Autodesk Inventor part; units mm, degrees
ref_plane "YZ Plane" through (0, 0, 0) normal (1, 0, 0) x (0, 1, 0)
ref_plane "XZ Plane" through (0, 0, 0) normal (0, 1, 0) x (-1, 0, 0)
ref_plane "XY Plane" through (0, 0, 0) normal (0, 0, 1) x (1, 0, 0)
sketch "Sketch1" plane through (0, 0, 0) normal (0, 1, 0) x (-1, 0, 0)
  line L0 (-75, 47.5) -> (75, 47.5)
  line L1 (75, 47.5) -> (75, -47.5)
  line L2 (75, -47.5) -> (-75, -47.5)
  line L3 (-75, -47.5) -> (-75, 47.5)
  line L4 (-75, 47.5) -> (75, -47.5) construction
  line L5 (75, 47.5) -> (-75, -47.5) construction
  point P0 (0, 0)
  dimension "d0" = 150
  dimension "d1" = 95
extrude "Extrusion1" add sketch "Sketch1" along normal blind 3
sketch "Sketch4" plane through (0, 3, 0) normal (0, 1, 0) x (1, 0, 0)
  line L0 (75, 47.5) -> (-75, 47.5)
  line L1 (-10, 47.5) -> (10, 47.5)
  line L2 (10, 47.5) -> (10, 27.5)
  line L3 (-10, 47.5) -> (-10, 27.5)
  line L4 (-10, 27.5) -> (10, 27.5)
  line L5 (-13, 47.5) -> (-7, 47.5)
  line L6 (7, 47.5) -> (13, 47.5)
  line L7 (-10, 47.5) -> (-10, 42.5)
  line L8 (10, 47.5) -> (10, 42.5)
  line L9 (-10, 42.5) -> (-10, 39.5)
  line L10 (10, 42.5) -> (10, 39.5)
  line L11 (-10, 27.5) -> (-10, 30.5)
  line L12 (10, 27.5) -> (10, 30.5)
  circle A0 centre (-10, 30.5) radius 3
  circle A1 centre (10, 30.5) radius 3
  circle A2 centre (-10, 39.5) radius 3
  circle A3 centre (10, 39.5) radius 3
  line L13 (-13, 39.5) -> (-13, 30.5)
  line L14 (-7, 39.5) -> (-7, 30.5)
  line L15 (7, 39.5) -> (7, 30.5)
  line L16 (13, 39.5) -> (13, 30.5)
  line L17 (-10, 27.5) -> (-7, 27.5)
  line L18 (-7, 27.5) -> (-7, 47.5)
  line L19 (-7, 47.5) -> (-10, 47.5)
  line L20 (-10, 47.5) -> (-10, 27.5)
  line L21 (-10, 47.5) -> (-13, 47.5)
  line L22 (-13, 47.5) -> (-13, 27.5)
  line L23 (-13, 27.5) -> (-10, 27.5)
  line L24 (-10, 27.5) -> (-10, 47.5)
  line L25 (10, 27.5) -> (7, 27.5)
  line L26 (7, 27.5) -> (7, 47.5)
  line L27 (7, 47.5) -> (10, 47.5)
  line L28 (10, 47.5) -> (10, 27.5)
  line L29 (10, 27.5) -> (13, 27.5)
  line L30 (13, 27.5) -> (13, 47.5)
  line L31 (13, 47.5) -> (10, 47.5)
  line L32 (10, 47.5) -> (10, 27.5)
  point P0 (0, 0)
  point P1 (0, 47.5)
  point P2 (7, 47.5)
  point P3 (7, 39.5)
  point P4 (-7, 39.5)
  point P5 (-7, 47.5)
  point P6 (-13, 47.5)
  point P7 (-13, 39.5)
  dimension "d14" = 20
  dimension "d15" = 20
  dimension "d16" = 6
  dimension "d17" = 6
  dimension "d18" = 5
  dimension "d19" = 5
  dimension "d20" = 3
  dimension "d21" = 3
  dimension "d22" = 3
  dimension "d23" = 3
extrude "Extrusion3" cut sketch "Sketch4" against normal through all contours A3 L2 | L16 A1 L2 A3 | L2 A3 | L2 A1 L15 A3 | A1 L2 | L2 A1 | A2 L3 | L14 A0 L3 A2 | L3 A2 | L3 A0 L13 A2 | A0 L3 | L3 A0
extrude "Extrusion5" cut sketch "Sketch4" against normal blind 1.2 contours L30 A3 L2 L0 | L2 A3 L26 L0 | L18 A2 L3 L0 | L3 A2 L22 L0
sketch "Sketch6" plane through (0, 3, 0) normal (0, 1, 0) x (1, 0, 0)
  line L0 (75, 47.5) -> (-75, 47.5)
  line L1 (0, 47.5) -> (0, 22.5)
  line L2 (0, 22.5) -> (0, -20.7)
  line L3 (0, -20.7) -> (0, 0.9)
  line L4 (0, 0.9) -> (-53.4, 0.9)
  line L5 (-53.4, -15.1) -> (-53.4, 16.9)
  circle A0 centre (-53.4, 16.9) radius 3
  circle A1 centre (-53.4, -15.1) radius 3
  line L6 (-19, 0.9) -> (19, 0.9)
  circle A2 centre (19, 0.9) radius 2.5
  circle A3 centre (-19, 0.9) radius 2.5
  line L7 (-19, 0.9) -> (-17, 0.9)
  line L8 (19, 0.9) -> (17, 0.9)
  circle A4 centre (17, 0.9) radius 2.5
  circle A5 centre (-17, 0.9) radius 2.5
  line L9 (-19, 3.4) -> (-17, 3.4)
  line L10 (-19, -1.6) -> (-17, -1.6)
  line L11 (17, 3.4) -> (19, 3.4)
  line L12 (17, -1.6) -> (19, -1.6)
  point P0 (0, 0)
  dimension "d40" = 25
  dimension "d41" = 43.2
  dimension "d42" = 53.4
  dimension "d43" = 32
  dimension "d44" = 6
  dimension "d45" = 6
  dimension "d46" = 38
  dimension "d47" = 5
  dimension "d48" = 5
  dimension "d49" = 2
  dimension "d50" = 2
  dimension "d51" = 5
  dimension "d52" = 5
extrude "Extrusion6" cut sketch "Sketch6" against normal through all
sketch "Sketch7" plane through (0, 3, 0) normal (0, 1, 0) x (1, 0, 0)
  line L0 (75, 47.5) -> (-75, 47.5)
  line L1 (-75, -47.5) -> (75, -47.5)
  line L2 (75, 47.5) -> (35, 47.5)
  line L3 (35, 47.5) -> (35, -47.5)
  line L4 (35, -47.5) -> (75, -47.5)
  line L5 (75, -47.5) -> (75, 47.5)
  point P0 (0, 0)
  point P1 (75, -47.5)
  dimension "d55" = 40
extrude "Extrusion7" cut sketch "Sketch7" against normal through all
sketch "Sketch8" plane through (0, 3, 0) normal (0, 1, 0) x (1, 0, 0)
  line L0 (-75, -47.5) -> (35, -47.5)
  line L1 (7, 47.5) -> (-7, 47.5)
  line L2 (0, 47.5) -> (0, -42.5)
  circle A0 centre (0, -42.5) radius 25
  circle A1 centre (0, -42.5) radius 20
  line L3 (0, -42.5) -> (-20, -42.5)
  circle A2 centre (-20, -42.5) radius 1.5
  circle A3 centre (-10, -59.8205) radius 1.5
  circle A4 centre (10, -59.8205) radius 1.5
  circle A5 centre (20, -42.5) radius 1.5
  circle A6 centre (10, -25.1795) radius 1.5
  circle A7 centre (-10, -25.1795) radius 1.5
  circle A8 centre (0, -42.5) radius 17
  line L4 (-17, -42.5) -> (-17, -47.5)
  line L5 (17, -42.5) -> (17, -47.5)
  point P0 (0, 0)
  dimension "d60" = 90
  dimension "d61" = 50
  dimension "d62" = 40
  dimension "d63" = 20
  dimension "d64" = 3
  dimension "d67" = 360
  dimension "d69" = 34
extrude "Extrusion8" cut sketch "Sketch8" against normal through all contours L4 A8 L0 | A2 A1 | A1 L3 A2 | A8 L3 L2 L0 | A8 L2 L3 | A1 A2 L3 | A6 A1 | A1 A6 | A7 A1 | A1 A7 | L0 A8 L5 | A5 A1 | A1 A5
fillet "Fillet1" radius 10 4 edges at (35, 1.5, 47.5) (35, 1.5, -47.5) (-75, 1.5, 47.5) (-75, 1.5, -47.5)
properties part number "TopMount"
Check sheet for the modelled part. Datum: model origin and axes. Units: mm. A direction names the side the tool comes from. Give positions to 0.01 mm unless a question says otherwise; leave off trailing zeros. Write each loop counter-clockwise with the first axis right and the second up, starting at its lowest first coordinate (ties: lowest second). Pieces come first, ordered by that corner, then holes. Notation, with made-up numbers: (87.25, 47.25) - (126.25, 47.25) arc R26 ccw to (126.25, 86.25) - close; hole circle Ø8 at (-36.5, -3). An arc over 180 degrees is marked (long way). Answer as a JSON object with one key per item and string values. Group by question number.
1) Access from +Z, -Z, +X, -X, +Y, -Y to the whole of each face (thin tool, end or side, straight path). Record for faces 1 (the face through (-14.5, 1.5, -0.8)), 2 (the face through (-7, 2, -37)), 3 (the face through (0.374, 1.521, 25.504)).
2) Thickness scan on probe 1 along X at (y, z) = (2.2, -1); probe 2 along X at (y, z) = (2.3, -16.9); probe 3 along Z at (x, y) = (-53.4, 1.5). Record the ranges inside material, lowest first. Write a range as from..to.
3) Sectioned sample at A-A (x = -53.4). Record the cut outline in (y, z).
4) Release check for a two-part mould opening along X. For faces 4 (the face through (20, 2, 44)), 5 (the face through (-71.99, 1.52, -44.65)), 6 (the face through (21, 1, 47.5)), 7 (the face through (-13, 2, -37)) record: pulls with the +X half, pulls with the -X half, needs draft (parallel to the pull), parting line crosses it, or undercut.
5) Sectioned sample at D-D (x = 0.5). Record the cut outline in (y, z).
6) Depth check by flat-ended pin: P1, Ø10, axis at x = 21, z = -15, coming from the -Y side; P2, Ø1.5, axis at y = 1.5, z = -38.5, coming from the +X side; P3, Ø3, axis at x = 10, z = -45, coming from the +Y side; P4, Ø5, axis at x = -53.4, z = -16.9, coming from the +Y side. Enter the tip coordinate at first touch or a pass-through.
7) Sectioned sample at B-B (z = 15.1). Record the cut outline in (x, y), then the cut area to 3 significant figures.
8) Sectioned sample at C-C (y = 0.7). Give the number of separate pieces and of enclosed holes in the cut face, then the cut area to 3 significant figures.
Geometry results:
{
 "1": {"face 1": "+Y, -Y", "face 2": "+Y", "face 3": "+Z, +Y, -Y"},
 "2": {"probe 1": "x = -75..-21.5, -14.5..14.5, 21.5..35", "probe 2": "x = -75..-56.4, -50.4..35", "probe 3": "z = -47.5..-19.9, -13.9..12.1, 18.1..47.5"},
 "3": {"outline": "(0, -47.5) - (3, -47.5) - (3, -19.9) - (0, -19.9) - close; (0, -13.9) - (3, -13.9) - (3, 12.1) - (0, 12.1) - close; (0, 18.1) - (3, 18.1) - (3, 47.5) - (0, 47.5) - close"},
 "4": {"face 4": "undercut", "face 5": "pulls with the -X half", "face 6": "needs draft", "face 7": "undercut"},
 "5": {"outline": "(0, -47.5) - (3, -47.5) - (3, 25.51) - (0, 25.51) - close"},
 "6": {"P1": "stops at y = 0", "P2": "stops at x = 35", "P3": "stops at y = 1.8", "P4": "passes through"},
 "7": {"outline": "(-75, 0) - (-56.4, 0) - (-56.4, 3) - (-75, 3) - close; (-50.4, 0) - (35, 0) - (35, 3) - (-50.4, 3) - close", "area": "312 mm^2"},
 "8": {"separate pieces": "1", "enclosed holes": "10", "area": "9,430 mm^2"}
}
